Geometry: see drawing. Coordinates: mm, zero at the bounding-box minimum. A direction names the side the tool comes from. Give positions to 0.01 mm unless a question says otherwise; leave off trailing zeros. Write each loop counter-clockwise with the first axis right and the second up, starting at its lowest first coordinate (ties: lowest second). Pieces come first, ordered by that corner, then holes. Notation, with made-up numbers: (32, -14.5) -> (69, -14.5) arc R19 cw to (69, 21.5) -> close; hole circle Ø7 at (47.5, 7). An arc over 180 degrees is marked (long way). Use one line per item in the form item = value. Start each with the question number.
(1) Draft query along Z for the marked faces 3 and 4. Return one class per face: pulls with the +Z half, pulls with the -Z half, needs draft (parallel to the pull), parting line crosses it, or undercut.
(2) Cut plane A-A, the plane x = 4. Output: boundary loops of the cut face in (y, z) (3 decimals), and give its area (3 significant figures).
(3) First-contact query: P1, Ø1.5, axis at x = 5.5, y = 6.5, coming from the +Z side; P2, Ø6, axis at y = 7.5, z = 21, coming from the -X side; P3, Ø2.5, axis at x = 2, z = 11, coming from the +Y side. Flat tips, straight axial feed; report the tip coordinate or a pass-through.
(4) Cut plane D-D, the plane z = 21.5. Output: boundary loops of the cut face in (x, y), and give its area (3 significant figures).
(5) Material intervals for line 1 along Y through (x, z) = (6.5, 15); line 2 along Z through (x, y) = (3.25, 7.5); line 3 along Z through (x, y) = (3.75, 9.75), sorted ascending. Write a range as from..to.
(6) Cut plane B-B, the plane z = 3.75. Output: boundary loops of the cut face in (x, y).
(7) Set-up query: the marked faces 1 and 2. Return all of +Z, -Z, +X, -X, +Y, -Y with unobstructed straight access to the full face (end or side cutting, diameter ignored); none if empty.
(8) Cut plane C-C, the plane y = 5.5. Output: boundary loops of the cut face in (x, z) (3 decimals).
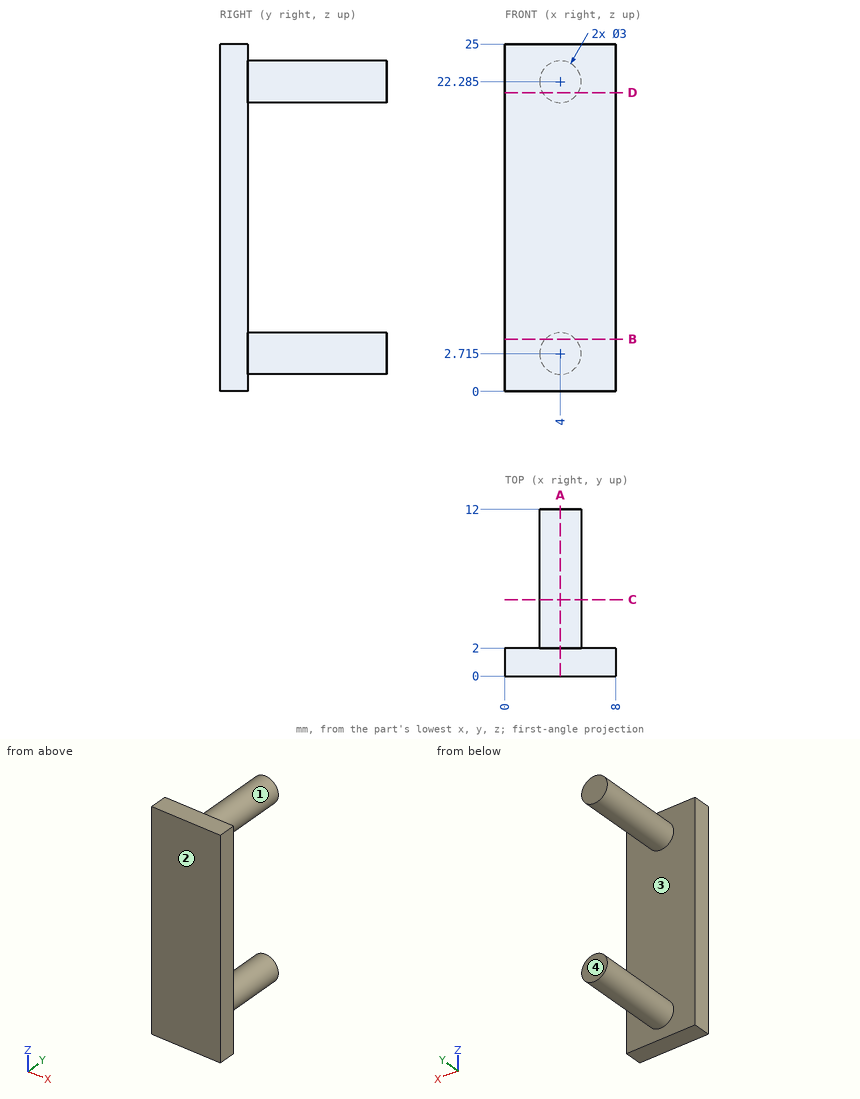
Geometry says:
q1.face_3 = undercut
q1.face_4 = needs draft
q2.outline = (0, 0) -> (2, 0) -> (2, 1.215) -> (12, 1.215) -> (12, 4.215) -> (2, 4.215) -> (2, 20.785) -> (12, 20.785) -> (12, 23.785) -> (2, 23.785) -> (2, 25) -> (0, 25) -> close
q2.area = 110 mm^2
q3.P1 = 23.58
q3.P2 = 2.5
q3.P3 = 2
q4.outline = (0, 0) -> (8, 0) -> (8, 2) -> (5.28, 2) -> (5.28, 12) -> (2.72, 12) -> (2.72, 2) -> (0, 2) -> close
q4.area = 41.6 mm^2
q5.line_1 = 0..2
q5.line_2 = 1.42..4.01, 20.99..23.58
q5.line_3 = 1.24..4.19, 20.81..23.76
q6.outline = (0, 0) -> (8, 0) -> (8, 2) -> (5.09, 2) -> (5.09, 12) -> (2.91, 12) -> (2.91, 2) -> (0, 2) -> close
q7.face_1 = +Y
q7.face_2 = +Z, -Z, +X, -X, -Y
q8.outline = circle Ø3 at (4, 2.715); circle Ø3 at (4, 22.285)
